Print and shaded views of the part. All mm, measured from the part's lowest x, y and z. Coordinates: 2 decimals unless noted, no trailing zeros. Loops run counter-clockwise (first coordinate to the right, second up) from the corner with the lowest first, then second, coordinate; pieces in that order, holes last. Notation, with made-up numbers: M 58.25,82 L 110.25,82 A24 cw 110.25,93 Z; hole C 45,-20.5 d3. An arc over 180 degrees is marked long. Answer as CSV lines item,"result". Start each with the question number.
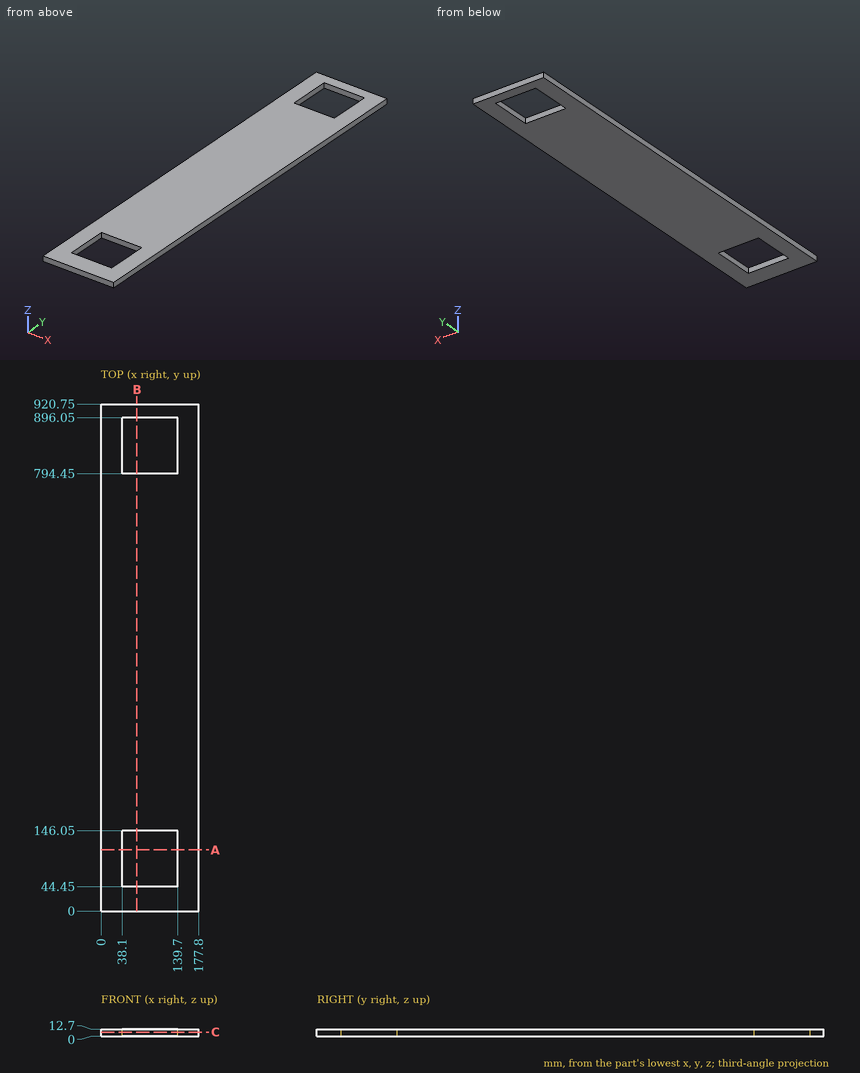
Q1. Slice it at B-B, the plane x = 65. Write the cut outline in (y, z), and give its area (3 significant figures).
Q2. Slice it at A-A, the plane y = 111. Write the cut outline in (x, z), and give its area (3 significant figures).
Q3. Wall check: L1, parallel to Y at x = 82, z = 9.25; L2, parallel to X at y = 842, z = 9.75. Give the ranges that are in metal, low to high.
Q4. Slice it at C-C, the plane z = 7. Write the cut outline in (x, y).
Solved:
1,outline,"M 0,0 L 44.45,0 L 44.45,12.7 L 0,12.7 Z; M 146.05,0 L 794.45,0 L 794.45,12.7 L 146.05,12.7 Z; M 896.05,0 L 920.75,0 L 920.75,12.7 L 896.05,12.7 Z"
1,area,"9,110 mm2"
2,outline,"M 0,0 L 38.1,0 L 38.1,12.7 L 0,12.7 Z; M 139.7,0 L 177.8,0 L 177.8,12.7 L 139.7,12.7 Z"
2,area,"968 mm2"
3,L1,"y = 0 to 44.45, 146.05 to 794.45, 896.05 to 920.75"
3,L2,"x = 0 to 38.1, 139.7 to 177.8"
4,outline,"M 0,0 L 177.8,0 L 177.8,920.75 L 0,920.75 Z; hole M 38.1,44.45 L 139.7,44.45 L 139.7,146.05 L 38.1,146.05 Z; hole M 38.1,794.45 L 139.7,794.45 L 139.7,896.05 L 38.1,896.05 Z"
